from build123d import *

# Parameters (mm, degrees)
F0_W      = 63
F0_H      = 7.7795209363
F1_DEPTH  = 29.1
F4_START  = 5
F3_W      = 73.4
F3_H      = 8.5
F4_DEPTH  = 34.9
F0_H_2    = 17.5400283188
F5_DEPTH  = 44.7
F6_R      = 1
F7_R      = 1.9
F8_DEPTH  = 12.9
F9_R      = 1.9
F10_DEPTH = 8.4
F11_START = -79.5
F11_DEPTH = 35.3


with BuildPart() as f1:
    # F0 (on Top) → F1 (new body)
    with BuildSketch(Plane.XY):
        Polygon((-31.5, 0), (-46.5, 0), (-46.5, -16), (46.5, -16), (46.5, 0), (31.5, 0), (31.5, -7.7795209363), (-31.5, -7.7795209363), align=None)
        with Locations((0, -3.8897604682)):
            Rectangle(F0_W, F0_H)
    extrude(amount=F1_DEPTH)

    # F3 (on line) → F4 (cut)
    with BuildSketch(Plane(origin=(0, -0.3915478696, 2.472135955), x_dir=(1, 0, 0), z_dir=(0, -0.156434465, 0.9876883406)).offset(F4_START)):
        with Locations((0, -4.75)):
            Rectangle(F3_W, F3_H)
    extrude(amount=F4_DEPTH, mode=Mode.SUBTRACT)

    # F0 (on Top) → F5 (cut)
    with BuildSketch(Plane.XY):
        with Locations((0, 8.7700141594)):
            Rectangle(F0_W, F0_H_2)
        with Locations((0, -3.8897604682)):
            Rectangle(F0_W, F0_H)
    extrude(amount=F5_DEPTH, mode=Mode.SUBTRACT)

    # F6
    f6_edges = [f1.edges().sort_by_distance(p)[0] for p in [
        (-39, 0, 29.1),
        (-31.5, -2.55761, 29.1),
        (-34.1, -5.11522, 29.1),
        (-36.7, -9.418197, 29.1),
        (0, -13.721173, 29.1),
        (36.7, -9.418197, 29.1),
        (34.1, -5.11522, 29.1),
        (31.5, -2.55761, 29.1),
        (39, 0, 29.1),
        (46.5, -8, 29.1),
        (0, -16, 29.1),
        (-46.5, -8, 29.1),
        (-46.5, 0, 14.55),
        (-46.5, -16, 14.55),
        (-46.5, -8, 0),
        (46.5, -16, 14.55),
        (0, -16, 0),
        (46.5, 0, 14.55),
        (46.5, -8, 0),
        (39, 0, 0),
        (31.5, 0, 14.55),
        (-31.5, 0, 14.55),
        (-39, 0, 0),
        (-31.5, -3.88976, 0),
        (0, -7.779521, 0),
        (31.5, -3.88976, 0),
    ]]
    fillet(f6_edges, radius=F6_R)

    # F7 (on face) → F8 (cut)
    with BuildSketch(Plane.YZ.offset(46.5)):
        with Locations((-4.75, 4.75)):
            Circle(F7_R)
    extrude(amount=-F8_DEPTH, mode=Mode.SUBTRACT)

    # F9 (on face) → F10 (cut)
    with BuildSketch(Plane.XZ.offset(16)):
        with Locations((41.75, 4.75)):
            Circle(F9_R)
        with Locations((-41.75, 4.75)):
            Circle(F9_R)
    extrude(amount=-F10_DEPTH, mode=Mode.SUBTRACT)

    # F7 (on face) → F11 (cut)
    with BuildSketch(Plane.YZ.offset(46.5).offset(F11_START)):
        with Locations((-4.75, 4.75)):
            Circle(F7_R)
    extrude(amount=-F11_DEPTH, mode=Mode.SUBTRACT)


solid = f1.part
Design review of the part built by this model. Coordinates are the model's own, in mm. A direction names the side the tool comes from. Coordinates: 2 decimals unless noted, no trailing zeros. Loops run counter-clockwise (first coordinate to the right, second up) from the corner with the lowest first, then second, coordinate; pieces in that order, holes last. Notation, with made-up numbers: (2.5, 52.25) - (34.5, 52.25) arc R28 ccw to (34.5, 87.25) - close; hole circle Ø11 at (-9, 36). An arc over 180 degrees is marked (long way). Use CSV: the item, a comma, the result in double quotes. Start each with the question number.
1. To check wall thickness, follow probe 1 along Z at (x, y) = (41.75, -13.5); probe 2 along X at (y, z) = (-8.25, 27.75); probe 3 along X at (y, z) = (-2, 12.75). State the ranges of each line that lie inside material, in increasing order.
2. Clearance check with flat-ended pins moving along their axes: pin 1 (2 mm diameter, centred on x = -28, z = 14, fed in from +Y); pin 2 (1.1 mm diameter, centred on x = -42.5, z = 4, fed in from -Y); pin 3 (4 mm diameter, centred on y = -4, z = 5.5, fed in from +X); pin 4 (4.5 mm diameter, centred on x = -10.5, z = 2.5, fed in from +Y). State where each tip first meets the part, or that it passes through.
3. Mouldability with a two-part tool opening along Z and no side actions: class faces 1 (the flat face through (-0.51, -11.8, 16.97)), 2 (the flat face through (-42, -7.6, 5)), 3 (the flat face through (-1, -16, 14)), 4 (the flat face through (42, -7.6, 5)) as released by +Z, released by -Z, zero draft, split by the parting line, or undercut.
4. For faces 5 (the cylindrical face through (-39.938, -11.859, 5.321)), 6 (the flat face through (-0.514, -8.605, 6.234)), 7 (the flat face through (31.5, -2, 11)), 8 (the flat face through (-39, 0, 14)), 9 (the cylindrical face through (-39.656, -6.15, 6.034)), list the 3-axis set-ups (+Z, -Z, +X, -X, +Y, -Y) from which the entire face can be reached by the end or side of a thin tool; tool diameter is ignored.
5. Add section D-D on x = -13.5. Give the boundary of the cut face in (y, z), plus the area to 3 significant figures.
6. Add section C-C on y = -12.5. Give the boundary of the cut face in (x, z), plus the area to 3 significant figures.
7. Add section A-A on x = -38.5. Give the boundary of the cut face in (y, z), plus the area to 3 significant figures.
Resolved:
1,probe 1,"0 to 2.85, 6.65 to 29.1"
1,probe 2,"-46.5 to -36.7, 36.7 to 46.5"
1,probe 3,"-46.5 to -31.5, 31.5 to 46.5"
2,pin 1,"y = -11.17"
2,pin 2,"y = -7.6"
2,pin 3,"x = 46.5"
2,pin 4,"y = -7.78"
3,face 1,"released by +Z"
3,face 2,"undercut"
3,face 3,"zero draft"
3,face 4,"undercut"
4,face 5,"-Y"
4,face 6,"none"
4,face 7,"+Z, -Z, +Y"
4,face 8,"+Z, -Z, +X, -X, +Y"
4,face 9,"-X"
5,outline,"(-16, 1) arc R1 ccw to (-15, 0) - (-8.78, 0) arc R1 ccw to (-7.78, 1) - (-7.78, 6.36) - (-10.06, 6) - (-13.59, 28.26) arc R1 ccw to (-14.58, 29.1) - (-15, 29.1) arc R1 ccw to (-16, 28.1) - close"
5,area,"144 mm2"
6,outline,"(-46.5, 1) arc R1 ccw to (-45.5, 0) - (45.5, 0) arc R1 ccw to (46.5, 1) - (46.5, 28.1) arc R1 ccw to (45.5, 29.1) - (37.7, 29.1) arc R1 ccw to (36.7, 28.1) - (36.7, 21.39) - (-36.7, 21.39) - (-36.7, 28.1) arc R1 ccw to (-37.7, 29.1) - (-45.5, 29.1) arc R1 ccw to (-46.5, 28.1) - close; hole circle Ø3.8 at (-41.75, 4.75); hole circle Ø3.8 at (41.75, 4.75)"
6,area,"2,120 mm2"
7,outline,"(-16, 1) arc R1 ccw to (-15, 0) - (-1, 0) arc R1 ccw to (0, 1) - (0, 28.1) arc R1 ccw to (-1, 29.1) - (-15, 29.1) arc R1 ccw to (-16, 28.1) - close; hole circle Ø3.8 at (-4.75, 4.75)"
7,area,"453 mm2"
